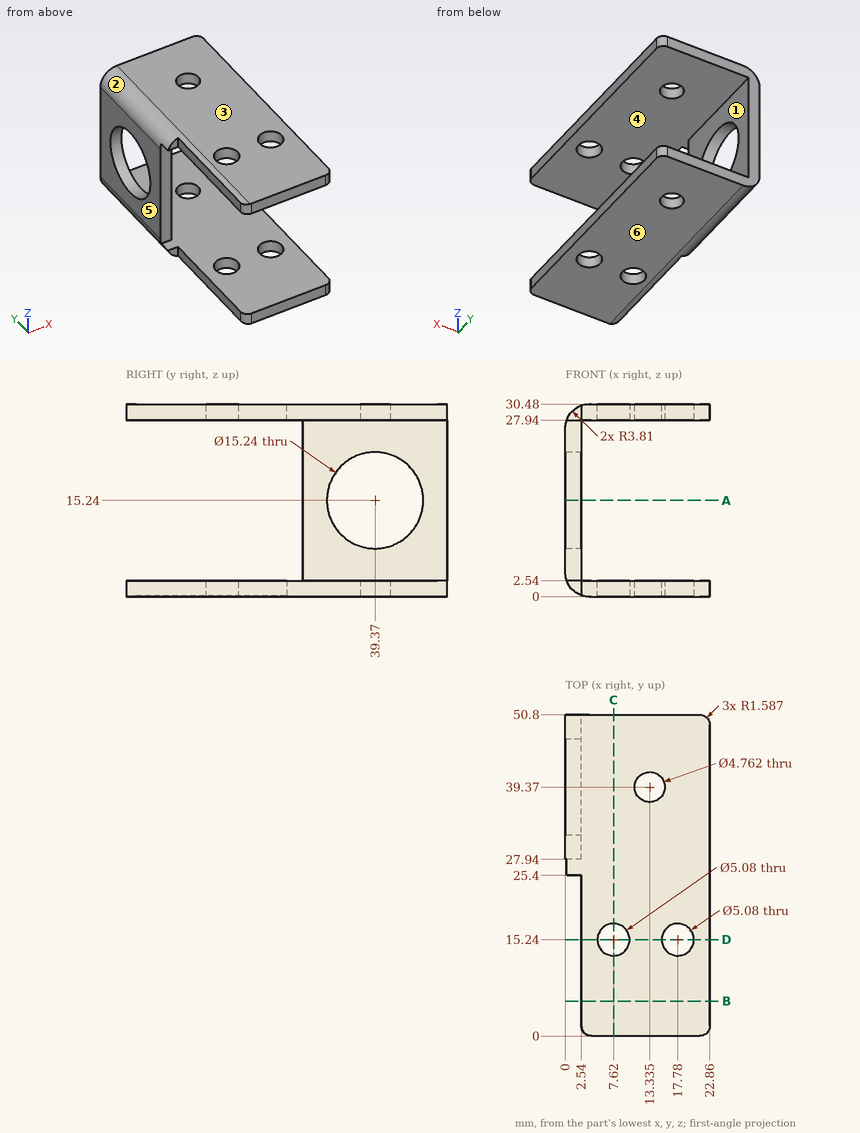
Geometry check sheet. Reference: drawing and pictorial views, mm from the part's lowest x, y, z. A direction names the side the tool comes from. Give positions to 0.01 mm unless a question says otherwise; leave off trailing zeros. Write each loop counter-clockwise with the first axis right and the second up, starting at its lowest first coordinate (ties: lowest second). Pieces come first, ordered by that corner, then holes. Notation, with made-up numbers: (36.25, 85.25) -> (65.25, 85.25) arc R24 ccw to (65.25, 97.25) -> close; hole circle Ø1 at (18, -13.75). An arc over 180 degrees is marked (long way). One line per item, written item: value. Start each with the question number.
Item 1: Section check A-A on z = 15.24. Record the cut outline in (x, y).
Item 2: Section check B-B on y = 5.5. Record the cut outline in (x, z), then the cut area to 3 significant figures.
Item 3: Material ranges on probe 1 along Z at (x, y) = (5.75, 44.5); probe 2 along X at (y, z) = (10, 2); probe 3 along X at (y, z) = (37, 3.5), recorded low to high. Write a range as from..to.
Item 4: Section check C-C on x = 7.62. Record the cut outline in (y, z).
Item 5: Gauge pin test, flat ends, axial feed: pin 1 (1.2 mm diameter, centred on x = 1.5, z = 1.5, fed in from -Y); pin 2 (1.2 mm diameter, centred on y = 10, z = 1, fed in from -X); pin 3 (0.8 mm diameter, centred on x = 1.5, z = 10.5, fed in from -Y). Record the tip position at first contact, or that the pin passes through.
Item 6: Section check D-D on y = 15.24. Record the cut outline in (x, z).
Item 7: Tool access check on the marked faces 1 and 2. Record the directions out of +Z, -Z, +X, -X, +Y, -Y that give a thin tool (end or side, any length) a straight path to the whole face; none if there is none.
Item 8: Draft check along Z on the marked faces 3, 4, 5 and 6. Enter one of: +Z half, -Z half, draft (parallel to the pull), parting line (faces both ways), or undercut.
Results list:
1. outline: (0, 27.94) -> (2.54, 27.94) -> (2.54, 31.75) -> (0, 31.75) -> close; (0, 46.99) -> (2.54, 46.99) -> (2.54, 50.8) -> (0, 50.8) -> close
2. outline: (2.54, 0.22) arc R3.81 ccw to (3.81, 0) -> (22.86, 0) -> (22.86, 2.54) -> (2.54, 2.54) -> close; (2.54, 27.94) -> (22.86, 27.94) -> (22.86, 30.48) -> (3.81, 30.48) arc R3.81 ccw to (2.54, 30.26) -> close
2. area: 103 mm²
3. probe 1: 0..2.54, 27.94..30.48
3. probe 2: 2.54..22.86
3. probe 3: 0.01..2.54
4. outline: (0, 0) -> (12.7, 0) -> (12.7, 2.54) -> (0, 2.54) -> close; (0, 27.94) -> (12.7, 27.94) -> (12.7, 30.48) -> (0, 30.48) -> close; (17.78, 0) -> (50.8, 0) -> (50.8, 2.54) -> (17.78, 2.54) -> close; (17.78, 27.94) -> (50.8, 27.94) -> (50.8, 30.48) -> (17.78, 30.48) -> close
5. pin 1: y = 25.4
5. pin 2: x = 2.54
5. pin 3: y = 27.94
6. outline: (2.54, 0.22) arc R3.81 ccw to (3.81, 0) -> (5.08, 0) -> (5.08, 2.54) -> (2.54, 2.54) -> close; (2.54, 27.94) -> (5.08, 27.94) -> (5.08, 30.48) -> (3.81, 30.48) arc R3.81 ccw to (2.54, 30.26) -> close; (10.16, 0) -> (15.24, 0) -> (15.24, 2.54) -> (10.16, 2.54) -> close; (10.16, 27.94) -> (15.24, 27.94) -> (15.24, 30.48) -> (10.16, 30.48) -> close; (20.32, 0) -> (22.86, 0) -> (22.86, 2.54) -> (20.32, 2.54) -> close; (20.32, 27.94) -> (22.86, 27.94) -> (22.86, 30.48) -> (20.32, 30.48) -> close
7. face 1: +X, +Y, -Y
7. face 2: +Z, -X, +Y, -Y
8. face 3: +Z half
8. face 4: undercut
8. face 5: draft
8. face 6: -Z half
